Check sheet for the modelled part. Datum: model origin and axes. Units: mm. A direction names the side the tool comes from. Coordinates: 2 decimals unless noted, no trailing zeros. Loops run counter-clockwise (first coordinate to the right, second up) from the corner with the lowest first, then second, coordinate; pieces in that order, holes last. Notation, with made-up numbers: M -2.5,88.5 L 34.5,88.5 A18 ccw 34.5,94.5 Z; hole C 25.25,25 d10. An arc over 180 degrees is marked long. Answer in a Markdown table with one row per item. Add a question column.
```python
from build123d import *

# Parameters (mm, degrees)
F0_W     = 76.2
F0_H     = 127
F1_DEPTH = 3.175
F2_W     = 38.1
F2_H     = 17.7633663237
F3_DEPTH = 3.175


# Not quite as in the source:
# - a length typed as a fraction of an inch, garbled in the dataset ("3 / 203.2 mm" for 3/8 in), is restored


with BuildPart() as f1:
    # F0 (on Top) → F1 (new body)
    with BuildSketch(Plane.XY):
        with Locations((-7.4443402648, 10.8384059966)):
            Rectangle(F0_W, F0_H)
    extrude(amount=F1_DEPTH)

    # F2 (on face) → F3 (cut)
    with BuildSketch(Plane(origin=(0, 0, 0), x_dir=(1, 0, 0), z_dir=(0, 0, -1))):
        with Locations((-7.4443402648, -62.2817228347)):
            Rectangle(F2_W, F2_H)
    extrude(amount=-F3_DEPTH, mode=Mode.SUBTRACT)


solid = f1.part
```
Q1. Access from +Z, -Z, +X, -X, +Y, -Y to the whole of each face (thin tool, end or side, straight path). Record for faces 1 (the face through (30.656, 10, 2)), 2 (the face through (-26.494, 62, 2)).
Q2. Mould release check, pull along Y, two halves, no side actions. Record for faces 3 (the face through (-8, 53.4, 2)), 4 (the face through (-8, 74.338, 2)), 5 (the face through (-8, 12, 0)): released by +Y, released by -Y, zero draft, split by the parting line, or undercut.
Q3. Cross-section at A-A (y = 58). Record the cut outline in (x, z) (3 decimals), plus the area to 3 significant figures.
Q4. Cross-section at C-C (z = 1.25). Record the cut outline in (x, y).
Q5. Thickness scan on L1, parallel to Y at x = -10, z = 2.2; L2, parallel to X at y = 62.5, z = 0.2. Record the ranges inside material, lowest first.
Q6. Go/stop test with a flat-tipped pin: pin 1 (6 mm diameter, centred on x = -14, y = 58.5, fed in from -Z). Record where the tip stops, or that it passes through.
Q7. Cross-section at B-B (x = 4.5). Record the cut outline in (y, z) (3 decimals), plus the area to 3 significant figures.
Answer key:
| question | item | result |
|---|---|---|
| 1 | face 1 | +Z, -Z, +X, +Y, -Y |
| 1 | face 2 | +Z, -Z |
| 2 | face 3 | undercut |
| 2 | face 4 | released by +Y |
| 2 | face 5 | zero draft |
| 3 | outline | M -45.544,0 L -26.494,0 L -26.494,3.175 L -45.544,3.175 Z; M 11.606,0 L 30.656,0 L 30.656,3.175 L 11.606,3.175 Z |
| 3 | area | 121 mm^2 |
| 4 | outline | M -45.54,-52.66 L 30.66,-52.66 L 30.66,74.34 L -45.54,74.34 Z; hole M -26.49,53.4 L 11.61,53.4 L 11.61,71.16 L -26.49,71.16 Z |
| 5 | L1 | -52.66 to 53.4, 71.16 to 74.34 |
| 5 | L2 | -45.54 to -26.49, 11.61 to 30.66 |
| 6 | pin 1 | through |
| 7 | outline | M -52.662,0 L 53.4,0 L 53.4,3.175 L -52.662,3.175 Z; M 71.163,0 L 74.338,0 L 74.338,3.175 L 71.163,3.175 Z |
| 7 | area | 347 mm^2 |
